from build123d import *

# Parameters (mm, degrees)
F0_W     = 22.28
F0_H     = 39.2
F1_DEPTH = 20
F2_R     = 4
F3_W     = 19.058216
F3_H     = 16.900683
F4_DEPTH = 24.2
F5_R     = 4
F6_R     = 4


with BuildPart() as f1:
    # F0 (on Top) → F1 (new body)
    with BuildSketch(Plane.XY):
        Rectangle(F0_W, F0_H)
    extrude(amount=F1_DEPTH)

    # F2
    f2_edges = [f1.edges().sort_by_distance(p)[0] for p in [
        (-11.14, -19.6, 10),
        (11.14, -19.6, 10),
    ]]
    fillet(f2_edges, radius=F2_R)

    # F3 (on face) → F4 (join)
    with BuildSketch(Plane(origin=(0, 19.6, 0), x_dir=(-1, 0, 0), z_dir=(0, 1, 0))):
        with Locations((0, 10.068494)):
            Rectangle(F3_W, F3_H)
    extrude(amount=F4_DEPTH)

    # F5
    f5_edges = [f1.edges().sort_by_distance(p)[0] for p in [
        (-9.529108, 31.7, 1.618153),
        (9.529108, 31.7, 1.618153),
        (-9.529108, 31.7, 18.518836),
        (9.529108, 31.7, 18.518836),
    ]]
    fillet(f5_edges, radius=F5_R)

    # F6
    f6_edges = [f1.edges().sort_by_distance(p)[0] for p in [
        (9.529108, 43.8, 10.068495),
        (0, 43.8, 18.518836),
        (-9.529108, 43.8, 10.068495),
        (0, 43.8, 1.618153),
    ]]
    fillet(f6_edges, radius=F6_R)


solid = f1.part
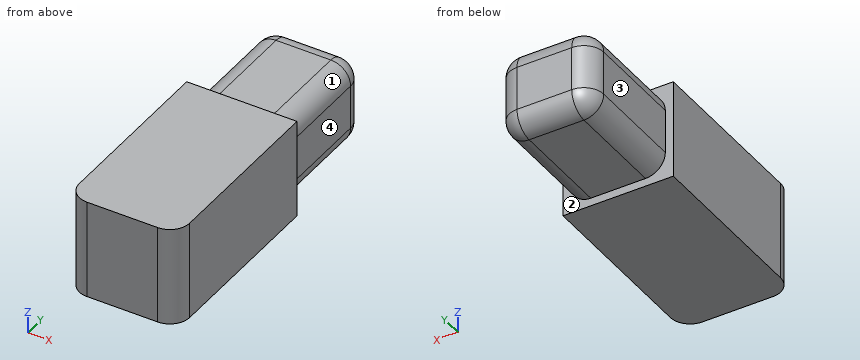
Design review of the part built by this model. Coordinates are the model's own, in mm. Face numbers are marked on the shaded views. A direction names the side the tool comes from. Coordinates: 2 decimals unless noted, no trailing zeros. Order: outer loops, then holes, each group sorted by start corner. A loop starts at its lowest first (then second) coordinate and runs counter-clockwise, first axis right, second up.
Item 1: Take a section at B-B, the plane y = 40.5. Write out the cut boundary in (x, z), then the cut area to 3 significant figures.
Item 2: For pin 1 Ø10 at (y, z) = (29, 11) entering from +X; pin 2 Ø4.5 at (y, z) = (30, 12) entering from -X; pin 3 Ø10 at (x, y) = (-8.5, 2) entering from -Z; pin 4 Ø3.5 at (x, y) = (1, 29.5) entering from +Z, all flat-tipped, find the tip position at first contact; note any pin that passes through.
Item 3: Take a section at A-A, the plane x = 1. Write out the cut boundary in (y, z), then the cut area to 3 significant figures.
Item 4: For the marked faces 1, 2, 3 and 4, list the 3-axis set-ups (+Z, -Z, +X, -X, +Y, -Y) from which the entire face can be reached by the end or side of a thin tool; tool diameter is ignored.
Item 5: For line 1 (Y direction, x = -4.75, z = 5.5); line 2 (Y direction, x = 0.5, z = 19.25); line 3 (X direction, y = 25, z = 8), list the stretches that pass through material, from the lowest coordinate up.
Item 6: Take a section at D-D, the plane z = 8.75. Write out the cut boundary in (x, y).
Item 7: Take a section at C-C, the plane z = 16.25. Write out the cut boundary in (x, y).
The answers:
1. outline: (-9.47, 5.62) arc R3.94 ccw to (-5.53, 1.68) - (5.53, 1.68) arc R3.94 ccw to (9.47, 5.62) - (9.47, 14.52) arc R3.94 ccw to (5.53, 18.46) - (-5.53, 18.46) arc R3.94 ccw to (-9.47, 14.52) - close
1. area: 304 mm2
2. pin 1: stops at x = 9.53
2. pin 2: stops at x = -9.53
2. pin 3: stops at z = 0
2. pin 4: stops at z = 18.52
3. outline: (-19.6, 0) - (19.6, 0) - (19.6, 1.62) - (39.8, 1.62) arc R4 ccw to (43.8, 5.62) - (43.8, 14.52) arc R4 ccw to (39.8, 18.52) - (19.6, 18.52) - (19.6, 20) - (-19.6, 20) - close
3. area: 1,190 mm2
4. face 1: +Z, +X, +Y
4. face 2: +Y
4. face 3: +Z, -Z, -X, +Y
4. face 4: +Z, -Z, +X, +Y
5. line 1: y = -19.6 to 43.8
5. line 2: y = -19.6 to 19.6
5. line 3: x = -9.53 to 9.53
6. outline: (-11.14, -15.6) arc R4 ccw to (-7.14, -19.6) - (7.14, -19.6) arc R4 ccw to (11.14, -15.6) - (11.14, 19.6) - (9.53, 19.6) - (9.53, 39.8) arc R4 ccw to (5.53, 43.8) - (-5.53, 43.8) arc R4 ccw to (-9.53, 39.8) - (-9.53, 19.6) - (-11.14, 19.6) - close
7. outline: (-11.14, -15.6) arc R4 ccw to (-7.14, -19.6) - (7.14, -19.6) arc R4 ccw to (11.14, -15.6) - (11.14, 19.6) - (9.14, 19.6) - (9.14, 39.8) arc R3.61 ccw to (5.53, 43.41) - (-5.53, 43.41) arc R3.61 ccw to (-9.14, 39.8) - (-9.14, 19.6) - (-11.14, 19.6) - close
